from build123d import *

# Parameters (mm, degrees)
F0_W     = 58.674
F0_H     = 123.698
F1_DEPTH = 7.62
F3_DEPTH = 0.508
F4_R     = 1.905
F5_DEPTH = 19.05
F6_R     = 0.635
F7_DEPTH = 0.508


with BuildPart() as f1:
    # F0 (on Front) → F1 (new body)
    with BuildSketch(Plane.XZ):
        with Locations((-29.337, 61.849)):
            Rectangle(F0_W, F0_H)
    extrude(amount=F1_DEPTH)

    # F2 (on face) → F3 (join)
    with BuildSketch(Plane.XY.offset(123.698)):
        with BuildLine():
            ThreePointArc((-15.494, -4.064), (-15.7915795103, -4.7824204897), (-16.51, -5.08))
            Line((-16.51, -5.08), (-7.62, -5.08))
            ThreePointArc((-7.62, -5.08), (-8.636, -4.064), (-7.62, -3.048))
            Line((-7.62, -3.048), (-16.51, -3.048))
            ThreePointArc((-16.51, -3.048), (-15.7915795103, -3.3455795103), (-15.494, -4.064))
        make_face()
        with BuildLine():
            ThreePointArc((-16.51, -3.048), (-17.526, -4.064), (-16.51, -5.08))
            Line((-16.51, -5.08), (-16.51, -3.048))
        make_face()
        with BuildLine():
            Line((-16.51, -3.048), (-16.51, -5.08))
            ThreePointArc((-16.51, -5.08), (-15.7915795103, -4.7824204897), (-15.494, -4.064))
            ThreePointArc((-15.494, -4.064), (-15.7915795103, -3.3455795103), (-16.51, -3.048))
        make_face()
        with BuildLine():
            ThreePointArc((-7.62, -3.048), (-8.636, -4.064), (-7.62, -5.08))
            Line((-7.62, -5.08), (-7.62, -3.048))
        make_face()
        with BuildLine():
            Line((-7.62, -3.048), (-7.62, -5.08))
            ThreePointArc((-7.62, -5.08), (-6.9015795103, -4.7824204897), (-6.604, -4.064))
            ThreePointArc((-6.604, -4.064), (-6.9015795103, -3.3455795103), (-7.62, -3.048))
        make_face()
    extrude(amount=F3_DEPTH)

    # F4 (on face) → F5 (cut)
    with BuildSketch(Plane(origin=(0, 0, 0), x_dir=(1, 0, 0), z_dir=(0, 0, -1))):
        with Locations((-47.244, 3.81)):
            Circle(F4_R)
    extrude(amount=-F5_DEPTH, mode=Mode.SUBTRACT)

    # F6 (on face) → F7 (cut)
    with BuildSketch(Plane(origin=(0, 0, 0), x_dir=(1, 0, 0), z_dir=(0, 0, -1))):
        with Locations((-43.434, 3.8100001402)):
            Circle(F6_R)
        with Locations((-12.7, 3.81)):
            Circle(F6_R)
        with Locations((-10.668, 3.81)):
            Circle(F6_R)
        with Locations((-8.636, 3.81)):
            Circle(F6_R)
        with Locations((-6.604, 3.81)):
            Circle(F6_R)
    extrude(amount=-F7_DEPTH, mode=Mode.SUBTRACT)


solid = f1.part
Geometry check sheet. Reference: the model listing, model coordinates, mm. A direction names the side the tool comes from. Coordinates: 2 decimals unless noted, no trailing zeros. Answer in a Markdown table with one row per item. Add a question column.
1) Release check for a two-part mould opening along X. For faces 1 (the flat face through (-58.674, -4, 61)), 2 (the flat face through (-30, -4, 123.698)), 3 (the cylindrical face through (-46.22, -5.416, 9.392)) record: +X half, -X half, draft (parallel to the pull), parting line (faces both ways), or undercut.
2) Gauge pin test, flat end, axial feed: P1, Ø2, axis at x = -43.434, y = -3.81, coming from the +Z side. Record the tip position at first contact, or that the pin passes through.
3) Material ranges on line 1 along Z through (x, y) = (-21.5, -5.25), recorded low to high. Write a range as [from, to].
4) Set-up check for faces 4 (the flat face through (-30, -4, 0)), 5 (the flat face through (-47, -4, 19.05)): record each of +Z, -Z, +X, -X, +Y, -Y from which the full face is reachable in a straight line by a thin tool's end or side.
Check result:
| question | item | result |
|---|---|---|
| 1 | face 1 | -X half |
| 1 | face 2 | draft |
| 1 | face 3 | undercut |
| 2 | P1 | stops at z = 123.7 |
| 3 | line 1 | z = [0, 123.7] |
| 4 | face 4 | -Z, +X, -X, +Y, -Y |
| 4 | face 5 | -Z |
